from build123d import *

# Parameters (mm, degrees)
SKETCH1_R           = 6.35
BOSS_EXTRUDE1_DEPTH = 596.9
SKETCH2_R           = 1.190625
CUT_EXTRUDE1_DEPTH  = 609.6
SKETCH6_OUTSIDE_W   = 134.134
SKETCH6_OUTSIDE_H   = 134.134
SKETCH6_OUTSIDE_R   = 5.9563
CUT_EXTRUDE2_DEPTH  = 0.635


with BuildPart() as part:
    # Sketch1 → Boss-Extrude1 (new body)
    with BuildSketch(Plane(origin=(0, 0, 0), x_dir=(1, 0, 0), z_dir=(0, 1, 0))):
        with Locations(Location((0, 0, 0), (0, 0, 270))):
            Circle(SKETCH1_R)
    extrude(amount=BOSS_EXTRUDE1_DEPTH)

    # Sketch2 → Cut-Extrude1 (cut)
    with BuildSketch(Plane(origin=(0, 596.9, 0), x_dir=(1, 0, 0), z_dir=(0, 1, 0))):
        with Locations(Location((0, 0, 0), (0, 0, 270))):
            Circle(SKETCH2_R)
    extrude(amount=-CUT_EXTRUDE1_DEPTH, mode=Mode.SUBTRACT)

    # Sketch6 outside → Cut-Extrude2 (cut)
    with BuildSketch(Plane(origin=(0, 95.25, 0), x_dir=(-1, 0, 0), z_dir=(0, -1, 0))):
        Rectangle(SKETCH6_OUTSIDE_W, SKETCH6_OUTSIDE_H)
        with Locations(Location((0, 0, 0), (0, 0, 90))):
            Circle(SKETCH6_OUTSIDE_R, mode=Mode.SUBTRACT)
    cut_extrude2 = extrude(amount=CUT_EXTRUDE2_DEPTH, mode=Mode.SUBTRACT)

    # Mirror1: Cut-Extrude2 across plane
    add(cut_extrude2.mirror(Plane(origin=(0, 298.45, 0), x_dir=(0, 0, 1), z_dir=(0, -1, 0))), mode=Mode.SUBTRACT)


solid = part.part
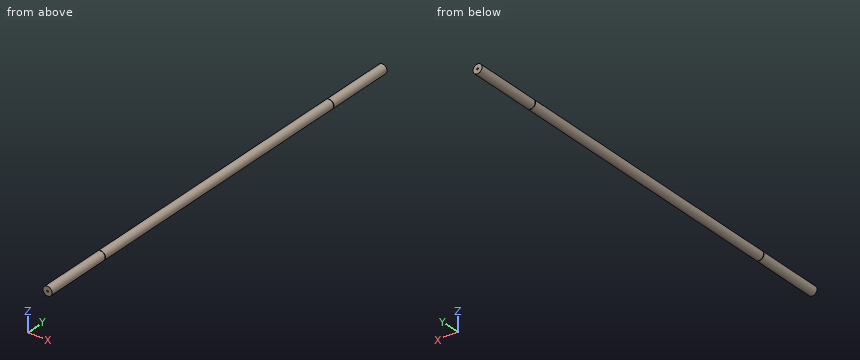
Source: CAD feature listing. Evaluate the final solid. Frame: model axes, mm. Coordinates: 2 decimals unless noted, no trailing zeros. Order: outer loops, then holes, each group sorted by start corner. A loop starts at its lowest first (then second) coordinate and runs counter-clockwise, first axis right, second up.
Item 1: Material intervals for line 1 (Y direction, x = 5.25, z = -3.25) (3 decimals); line 2 (Z direction, x = 0.25, y = 503.5); line 3 (X direction, y = 387, z = 0.5), sorted ascending.
Output values:
line 1: y = 0 to 94.615, 95.25 to 501.65, 502.285 to 596.9
line 2: z = -6.35 to -1.16, 1.16 to 6.35
line 3: x = -6.33 to -1.08, 1.08 to 6.33
Item 2: Cut plane A-A (y = 276). Return loops of the section in (x, z), plus the area to 3 significant figures.
Output values:
outline: circle Ø12.7 at (0, 0); hole circle Ø2.38 at (0, 0)
area: 122 mm2
Item 3: First-contact query: P1, Ø1.5, axis at y = 91, z = 1, coming from the +X side; P2, Ø3, axis at x = -2.5, y = 177, coming from the -Z side; P3, Ø3, axis at x = -2.5, y = 434.5, coming from the +Z side. Flat tips, straight axial feed; report the tip coordinate or a pass-through.
Output values:
P1: stops at x = 6.35
P2: stops at z = -6.27
P3: stops at z = 6.27
